from build123d import *

# Parameters (mm, degrees)
SCHIZZO1_R                   = 1.897864919
ESTRUSIONE_ESTRUSIONE1_DEPTH = 3.8
SCHIZZO7_W                   = 8
SCHIZZO7_H                   = 50
TAGLIO_ESTRUSIONE4_DEPTH     = 3.8
ESTRUSIONE_ESTRUSIONE4_DEPTH = 3.8
RACCORDO2_R                  = 1
SCHIZZO10_R                  = 3.5
TAGLIO_ESTRUSIONE5_DEPTH     = 10
TAGLIO_ESTRUSIONE6_DEPTH     = 1.5


with BuildPart() as part:
    # Schizzo1 → Estrusione-Estrusione1 (new body)
    with BuildSketch(Plane.XY):
        with BuildLine():
            Line((-4, 0), (-4, 80))
            ThreePointArc((-4, 80), (0, 84), (4, 80))
            Line((4, 80), (4, 0))
            ThreePointArc((4, 0), (0, -4), (-4, 0))
        make_face()
        with Locations(Location((0, 80, 0), (0, 0, 180))):
            Circle(SCHIZZO1_R, mode=Mode.SUBTRACT)
    extrude(amount=ESTRUSIONE_ESTRUSIONE1_DEPTH)

    # Schizzo7 → Taglio-Estrusione4 (cut)
    with BuildSketch(Plane.XY.offset(3.8)):
        with Locations((0, 21)):
            Rectangle(SCHIZZO7_W, SCHIZZO7_H)
    extrude(amount=-TAGLIO_ESTRUSIONE4_DEPTH, mode=Mode.SUBTRACT)

    # Schizzo9 → Estrusione-Estrusione4 (add)
    with BuildSketch(Plane.XY.offset(3.8)):
        with BuildLine():
            Line((-4, 46), (4, 46))
            ThreePointArc((4, 46), (-2.243289818, 22.859693708), (-19.27864045, 6))
            ThreePointArc((-19.27864045, 6), (-7.949658462, 24.590674614), (-4, 46))
        make_face()
    extrude(amount=-ESTRUSIONE_ESTRUSIONE4_DEPTH)

    # Raccordo2
    raccordo2_edges = [part.edges().sort_by_distance(p)[0] for p in [
        (-19.27864045, 6, 1.9),
    ]]
    fillet(raccordo2_edges, radius=RACCORDO2_R)

    # Schizzo10 → Taglio-Estrusione5 (cut)
    with BuildSketch(Plane.XY.offset(3.8)):
        with Locations((0, 80)):
            Circle(SCHIZZO10_R)
    extrude(amount=-TAGLIO_ESTRUSIONE5_DEPTH, mode=Mode.SUBTRACT)

    # Schizzo13 → Taglio-Estrusione6 (cut)
    with BuildSketch(Plane.XY.offset(3.8)):
        with BuildLine():
            Line((-2.75, 77.834936491), (-1.9, 65.9))
            ThreePointArc((-1.9, 65.9), (0, 64), (1.9, 65.9))
            Line((1.9, 65.9), (2.75, 77.834936491))
            ThreePointArc((2.75, 77.834936491), (1.145643924, 83.307189139), (-3.5, 80))
            ThreePointArc((-3.5, 80), (-3.307189139, 78.854356076), (-2.75, 77.834936491))
        make_face()
    extrude(amount=-TAGLIO_ESTRUSIONE6_DEPTH, mode=Mode.SUBTRACT)


solid = part.part
For this review, take the finished solid that the model builds, in its own axes (mm). A direction names the side the tool comes from. Round coordinates to 2 decimals unless told otherwise and drop trailing zeros. Write each loop counter-clockwise with the first axis right and the second up, starting at its lowest first coordinate (ties: lowest second). Pieces come first, ordered by that corner, then holes. Notation, with made-up numbers: M 62,42.5 L 108,42.5 A26 ccw 108,66.5 Z; hole C -39.75,18 d1. An arc over 180 degrees is marked long. Write item = value, one per line. Start each with the question number.
(1) We need section C-C (y = 67). Give the boundary of the cut face in (x, z), then the cut area to 3 significant figures.
(2) Clearance check with flat-ended pins moving along their axes: pin 1 Ø2 at (y, z) = (51, 3) entering from -X; pin 2 Ø8 at (x, y) = (-12, 27.5) entering from +Z. State where each tip first meets the part, or that it passes through.
(3) We need section B-B (y = 53.5). Give the boundary of the cut face in (x, z), then the cut area to 3 significant figures.
(4) We need section A-A (x = 0). Give the boundary of the cut face in (y, z), then the cut area to 3 significant figures.
(5) For faces 1 (the face through (4, 63, 2)), 2 (the face through (-4, 63, 2)), 3 (the face through (0, 71, 2.3)), list the 3-axis set-ups (+Z, -Z, +X, -X, +Y, -Y) from which the entire face can be reached by the end or side of a thin tool; tool diameter is ignored.
(6) The part is to be moulded in two halves that separate along Y. For faces 4 (the face through (0, 64, 3)), 5 (the face through (-6.97, 27.36, 1.93)), 6 (the face through (-3.5, 44.1, 3.8)), say which applies: +Y half, -Y half, draft (parallel to the pull), parting line (faces both ways), or undercut.
(7) We need section D-D (x = -8.25). Give the boundary of the cut face in (y, z), then the cut area to 3 significant figures.
(8) For line 1 along X through (y, z) = (80, 1.4); line 2 along Y through (x, z) = (0, 2.5); line 3 along X through (y, z) = (50, 0.75), list the stretches that pass through material, from the lowest coordinate up.
Results found:
q1.outline = M -4,0 L 4,0 L 4,3.8 L 1.98,3.8 L 1.98,2.3 L -1.98,2.3 L -1.98,3.8 L -4,3.8 Z
q1.area = 24.5 mm²
q2.pin_1 = -4
q2.pin_2 = through
q3.outline = M -4,0 L 4,0 L 4,3.8 L -4,3.8 Z
q3.area = 30.4 mm²
q4.outline = M 27.24,0 L 76.5,0 L 76.5,2.3 L 64,2.3 L 64,3.8 L 27.24,3.8 Z; M 83.5,0 L 84,0 L 84,3.8 L 83.5,3.8 Z
q4.area = 170 mm²
q5.face_1 = +Z, -Z, +X, +Y, -Y
q5.face_2 = +Z, -Z, -X, +Y
q5.face_3 = +Z
q6.face_4 = undercut
q6.face_5 = +Y half
q6.face_6 = draft
q7.outline = M 14.74,0 L 23.82,0 L 23.82,3.8 L 14.74,3.8 Z
q7.area = 34.5 mm²
q8.line_1 = -4 to -3.5, 3.5 to 4
q8.line_2 = 27.24 to 64, 83.5 to 84
q8.line_3 = -4 to 4
